The listing builds one solid part. Answer for the finished solid, in the listing's coordinates (mm). Face numbers are marked on the shaded views. A direction names the side the tool comes from. Coordinates: 2 decimals unless noted, no trailing zeros. Order: outer loops, then holes, each group sorted by start corner. A loop starts at its lowest first (then second) coordinate and runs counter-clockwise, first axis right, second up. Notation, with made-up numbers: (63, -6.5) - (101, -6.5) arc R18 ccw to (101, 19.5) - close; hole circle Ø6 at (-0.5, -29). An arc over 180 degrees is marked (long way). Use one line per item in the form item = value. Start each with the question number.
Item 1: Each of these flat-tipped pins is pushed along its axis until it touches: pin 1 Ø14.5 at (x, y) = (32.5, 0) entering from +Z; pin 2 Ø8 at (x, y) = (31.5, -4) entering from +Z; pin 3 Ø9 at (x, y) = (-1.5, -1) entering from +Z; pin 4 Ø5 at (y, z) = (-7.5, 22) entering from -X. Where does it stop, or does it pass through?
Item 2: Consider line 1 along Z through (x, y) = (0, 10.75); line 2 along Y through (x, z) = (32.5, 8.25); line 3 along Y through (x, z) = (32.5, 29). Determine where each line is inside the solid, lowest interval first. Write a range as [from, to].
Item 3: Section B-B, the plane y = 0 is taken. Count the separate pieces of the cut face and the enclosed holes in it, and give its area (3 significant figures).
Item 4: Section A-A, the plane z = 23 is taken. Write down the section's boundary in (x, y).
Item 5: A tool of negligible diameter and unlimited length cuts with its end or side. For the marked faces 5, 6 and 7, from which of +Z, -Z, +X, -X, +Y, -Y can it reach the whole face along a straight path? Write none if from no direction.
Item 6: Section C-C, the plane z = 27 is taken. Write down the section's boundary in (x, y), and give its area (3 significant figures).
Item 7: The mould has two halves that part along X. Classify the marked faces 1, 2, 3 and 4: released by +X, released by -X, zero draft, split by the parting line, or undercut.
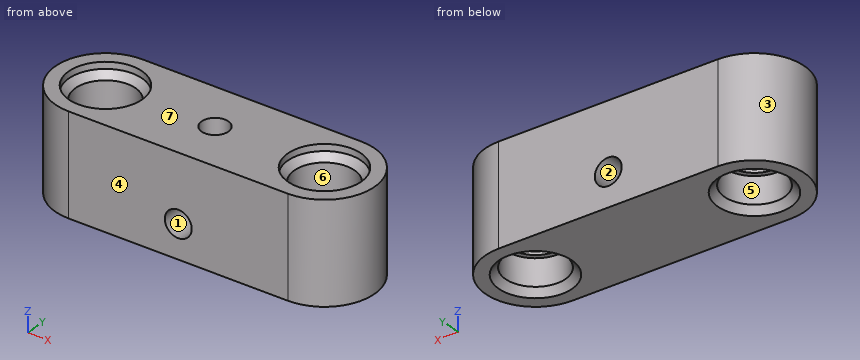
Autodesk Inventor part; units mm, degrees
ref_plane "YZ Plane" through (0, 0, 0) normal (1, 0, 0) x (0, 1, 0)
ref_plane "XZ Plane" through (0, 0, 0) normal (0, 1, 0) x (-1, 0, 0)
ref_plane "XY Plane" through (0, 0, 0) normal (0, 0, 1) x (1, 0, 0)
sketch "Náčrt1" plane through (0, 0, 0) normal (0, 0, 1) x (1, 0, 0)
  line L0 (-32.5, -15) -> (32.5, -15)
  line L1 (47.5, 0) -> (47.5, 0)
  line L2 (32.5, 15) -> (-32.5, 15)
  line L3 (-47.5, 0) -> (-47.5, 0)
  line L4 (-47.5, -15) -> (47.5, 15) construction
  line L5 (47.5, -15) -> (-47.5, 15) construction
  arc A0 (-32.5, 15) -> (-47.5, 0) centre (-32.5, 0) ccw
  arc A1 (-47.5, 0) -> (-32.5, -15) centre (-32.5, 0) ccw
  arc A2 (32.5, -15) -> (47.5, 0) centre (32.5, 0) ccw
  arc A3 (47.5, 0) -> (32.5, 15) centre (32.5, 0) ccw
  point P0 (0, 0)
  point P1 (47.5, 0)
  point P2 (-47.5, 0)
  dimension "d0" = 95
  dimension "d1" = 30
  dimension "d2" = 15
extrude "Vysunutí1" add sketch "Náčrt1" along normal blind 30
sketch "Náčrt2" plane through (0, 0, 30) normal (0, 0, 1) x (1, 0, 0)
  arc A0 (32.5, -15) -> (32.5, 15) centre (32.5, 0) ccw
  line L0 (32.5, 15) -> (-32.5, 15)
  arc A1 (-32.5, 15) -> (-32.5, -15) centre (-32.5, 0) ccw
  line L1 (-32.5, -15) -> (32.5, -15)
  point P0 (0, 0)
hole "Díra1" at (-32.5, 0, 30) at (32.5, 0, 30) direction (0, 0, -1) diameter 15 end through all
sketch "Náčrt3" plane through (0, 0, 30) normal (0, 0, 1) x (1, 0, 0)
  circle A0 centre (-32.5, 0) radius 7.5
  circle A1 centre (32.5, 0) radius 7.5
  circle A2 centre (-32.5, 0) radius 11
  circle A3 centre (32.5, 0) radius 11
  point P0 (0, 0)
  dimension "d14" = 22
  dimension "d15" = 22
extrude "Vysunutí2" cut sketch "Náčrt3" against normal blind 2 contours A1 | A2 | A3
sketch "Náčrt4" plane through (-32.5, 0, 28) normal (0, 0, 1) x (1, 0, 0)
  circle A0 centre (0, 0) radius 11
  circle A1 centre (0, 0) radius 7.5
  circle A2 centre (65, 0) radius 7.5
  circle A3 centre (0, 0) radius 9
  circle A4 centre (65, 0) radius 9
  point P0 (32.5, 0)
  dimension "d18" = 18
  dimension "d19" = 18
extrude "Vysunutí3" cut sketch "Náčrt4" against normal blind 17 contours A3 | A4
sketch "Náčrt5" plane through (0, 0, 0) normal (0, 0, -1) x (-1, 0, 0)
  circle A0 centre (32.5, 0) radius 7.5
  circle A1 centre (-32.5, 0) radius 7.5
  circle A2 centre (32.5, 0) radius 9
  circle A3 centre (-32.5, 0) radius 9
  point P0 (0, 0)
  dimension "d22" = 18
  dimension "d23" = 18
extrude "Vysunutí4" cut sketch "Náčrt5" against normal blind 10
chamfer "Zkosení1" distance 2 angle 45 4 edges at (-23.5, 0, 0) (41.5, 0, 0) (-41.5, 0, 28) (23.5, 0, 28)
sketch "Náčrt6" plane through (0, 0, 30) normal (0, 0, 1) x (1, 0, 0)
  circle A0 centre (0, 0) radius 4
  dimension "d29" = 8
extrude "Vysunutí5" cut sketch "Náčrt6" against normal blind 23
sketch "Náčrt7" plane through (-32.5, -15, 0) normal (0, -1, 0) x (1, 0, 0)
  circle A0 centre (32.5, 10) radius 4
  line L0 (0, 30) -> (65, 30)
  line L1 (0, 0) -> (65, 0)
  point P0 (32.5, 0)
  point P1 (32.5, 0)
  dimension "d32" = 8
  dimension "d33" = 20
extrude "Vysunutí6" cut sketch "Náčrt7" against normal blind 9
mirror "Zrcadlit1" about plane through (0, 0, 0) normal (0, 1, 0) of "Vysunutí6"
properties part number "P2 lmao fila" material "Ocel"
Response:
q1.pin_1 = through
q1.pin_2 = 11
q1.pin_3 = 30
q1.pin_4 = -46.64
q2.line_1 = [0, 6], [14, 30]
q2.line_2 = [-15, -9], [9, 15]
q2.line_3 = [-15, -11], [11, 15]
q3.separate_pieces = 3
q3.enclosed_holes = 0
q3.area = 1,560 mm2
q4.outline = (-32.5, -15) - (32.5, -15) arc R15 ccw to (32.5, 15) - (-32.5, 15) arc R15 ccw to start; hole circle Ø18 at (-32.5, 0); hole circle Ø8 at (0, 0); hole circle Ø18 at (32.5, 0)
q5.face_5 = -Z
q5.face_6 = +Z
q5.face_7 = +Z, +X, -X, +Y, -Y
q6.outline = (-32.5, -15) - (32.5, -15) arc R15 ccw to (32.5, 15) - (-32.5, 15) arc R15 ccw to start; hole circle Ø20 at (-32.5, 0); hole circle Ø8 at (0, 0); hole circle Ø20 at (32.5, 0)
q6.area = 1,980 mm2
q7.face_1 = undercut
q7.face_2 = undercut
q7.face_3 = released by -X
q7.face_4 = zero draft
